The model under review builds one solid part; all positions refer to its coordinate system, in mm. Give positions to 0.01 mm unless a question says otherwise; leave off trailing zeros. Loops run counter-clockwise (first coordinate to the right, second up) from the corner with the lowest first, then second, coordinate; pieces in that order, holes last. Notation, with made-up numbers: M 74.5,-29 L 119.5,-29 A17 ccw 119.5,-17 Z; hole C 12,-15.75 d7. An arc over 180 degrees is marked long. One line per item, written item: value. Start each with the question number.
Q1. For pin 1 (1 mm diameter, centred on x = -0.5, z = 72, fed in from -Y), flat-tipped, find the tip position at first contact; note if it passes through.
Q2. To check wall thickness, follow line 1 along Y through (x, z) = (-0.15, 22); line 2 along X through (y, z) = (0.85, 36). State the ranges of each line that lie inside material, in increasing order. Write a range as from..to.
Q3. We need section A-A on z = 18. Write out the cut boundary in (x, y), plus the area to 3 significant figures.
```python
from build123d import *

# Parameters (mm, degrees)
SKETCH_1_R      = 2.5
EXTRUDE_1_DEPTH = 135
CHAMFER_1_SIZE  = 0.2
SCALE_1_SCALE   = 0.6


with BuildPart() as part:
    # 草图1 → 凸台-拉伸1 (new body)
    with BuildSketch(Plane.XY):
        Circle(SKETCH_1_R)
    extrude(amount=EXTRUDE_1_DEPTH)

    # 倒角1
    chamfer_1_edges = [part.edges().sort_by_distance(p)[0] for p in [
        (-2.5, 0, 0),
        (-2.5, 0, 135),
    ]]
    chamfer(chamfer_1_edges, length=CHAMFER_1_SIZE)


with BuildPart() as part_1:
    # 缩放比例1: scaled about (0, 0, 0)
    add(part.part.scale(SCALE_1_SCALE))


solid = part_1.part
```
Solved:
1. pin 1: y = -1.5
2. line 1: -1.49..1.49
2. line 2: -1.24..1.24
3. outline: C 0,0 d3
3. area: 7.07 mm2
